```python
from build123d import *

# Parameters (mm, degrees)
SKETCH1_R           = 43.5
SKETCH1_R_2         = 37.5
EXTRUDE_THIN3_DEPTH = 31
FILLET5_R           = 3
FILLET6_R           = 1
SHELL4_START        = 5
SHELL4_OUTLINE_R    = 38.5
SHELL4_OUTLINE_R_2  = 37.5
SHELL4_DEPTH        = 21


# Read off the part's stored shape, not the designer's step: Shell4
with BuildPart() as part:
    # Sketch1 → Extrude-Thin3 (new body)
    with BuildSketch(Plane.XY):
        Circle(SKETCH1_R)
        Circle(SKETCH1_R_2, mode=Mode.SUBTRACT)
    extrude(amount=EXTRUDE_THIN3_DEPTH)

    # Fillet5
    fillet5_edges = [part.edges().sort_by_distance(p)[0] for p in [
        (-43.5, 0, 0),
        (-43.5, 0, 31),
    ]]
    fillet(fillet5_edges, radius=FILLET5_R)

    # Fillet6
    fillet6_edges = [part.edges().sort_by_distance(p)[0] for p in [
        (-37.5, 0, 0),
        (-37.5, 0, 31),
    ]]
    fillet(fillet6_edges, radius=FILLET6_R)

    # Shell4 outline → Shell4 (cut)
    with BuildSketch(Plane.XY.offset(SHELL4_START)):
        Circle(SHELL4_OUTLINE_R)
        Circle(SHELL4_OUTLINE_R_2, mode=Mode.SUBTRACT)
    extrude(amount=SHELL4_DEPTH, mode=Mode.SUBTRACT)


solid = part.part
```
Check sheet for the modelled part. Datum: model origin and axes. Units: mm. A direction names the side the tool comes from. Give positions to 0.01 mm unless a question says otherwise; leave off trailing zeros. Order: outer loops, then holes, each group sorted by start corner. A loop starts at its lowest first (then second) coordinate and runs counter-clockwise, first axis right, second up. Notation, with made-up numbers: (-4.75, 82) -> (1.25, 82) arc R32 ccw to (1.25, 112) -> close; hole circle Ø5 at (65.5, -15.5). An arc over 180 degrees is marked (long way). Return JSON: item names as keys, results as strings.
1. Go/stop test with flat-tipped pins: P1, Ø1.5, axis at x = -29, z = 6, coming from the -Y side; P2, Ø1, axis at y = -17, z = 15.5, coming from the +X side; P3, Ø2, axis at x = 31, z = 16.5, coming from the -Y side. Record where each tip stops, or that it passes through.
From the geometry:
{"P1": "y = -33.08", "P2": "x = 40.25", "P3": "y = -31.5"}
2. Mould release check, pull along X, two halves, no side actions. Record for faces 3 (the flat face through (36, -15, 31)), 4 (the flat face through (8, -37, 5)), 5 (the cylindrical face through (-5.66, 43.13, 15.32)): +X half, -X half, draft (parallel to the pull), parting line (faces both ways), or undercut.
From the geometry:
{"face 3": "draft", "face 4": "undercut", "face 5": "parting line"}
3. Cross-section at A-A, the plane y = 0. Record the cut outline in (x, z).
From the geometry:
{"outline": "(-43.5, 3) arc R3 ccw to (-40.5, 0) -> (-38.5, 0) arc R1 ccw to (-37.5, 1) -> (-37.5, 5) -> (-38.5, 5) -> (-38.5, 26) -> (-37.5, 26) -> (-37.5, 30) arc R1 ccw to (-38.5, 31) -> (-40.5, 31) arc R3 ccw to (-43.5, 28) -> close; (37.5, 1) arc R1 ccw to (38.5, 0) -> (40.5, 0) arc R3 ccw to (43.5, 3) -> (43.5, 28) arc R3 ccw to (40.5, 31) -> (38.5, 31) arc R1 ccw to (37.5, 30) -> (37.5, 26) -> (38.5, 26) -> (38.5, 5) -> (37.5, 5) -> close"}
4. Set-up check for faces 1 (the flat face through (36, -15, 0)), 2 (the cylindrical face through (-30.55, -23.43, 15.35)): record each of +Z, -Z, +X, -X, +Y, -Y from which the full face is reachable in a straight line by a thin tool's end or side.
From the geometry:
{"face 1": "-Z, +X, -X, +Y, -Y", "face 2": "none"}
5. Material ranges on probe 1 along Y at (x, z) = (0, 4); probe 2 along X at (y, z) = (-2, 30); probe 3 along X at (y, z) = (6, 23), recorded low to high. Write a range as [from, to].
From the geometry:
{"probe 1": "[-43.5, -37.5], [37.5, 43.5]", "probe 2": "[-42.69, -37.45], [37.45, 42.69]", "probe 3": "[-43.08, -38.03], [38.03, 43.08]"}
6. Cross-section at C-C, the plane z = 17. Record the cut outline in (x, y), plus the area to 3 significant figures.
From the geometry:
{"outline": "circle Ø87 at (0, 0); hole circle Ø77 at (0, 0)", "area": "1,290 mm^2"}
